Source: three-view drawing plus pictorial views. Frame: mm from the lowest corner of the part. A direction names the side the tool comes from. Give positions to 0.01 mm unless a question says otherwise; leave off trailing zeros. Write each loop counter-clockwise with the first axis right and the second up, starting at its lowest first coordinate (ties: lowest second). Pieces come first, ordered by that corner, then holes. Notation, with made-up numbers: M -22,87 L 31,87 A18 ccw 31,115 Z; hole C 20,35 d6. An arc over 180 degrees is marked long. One line per question, with ' | ' between items.
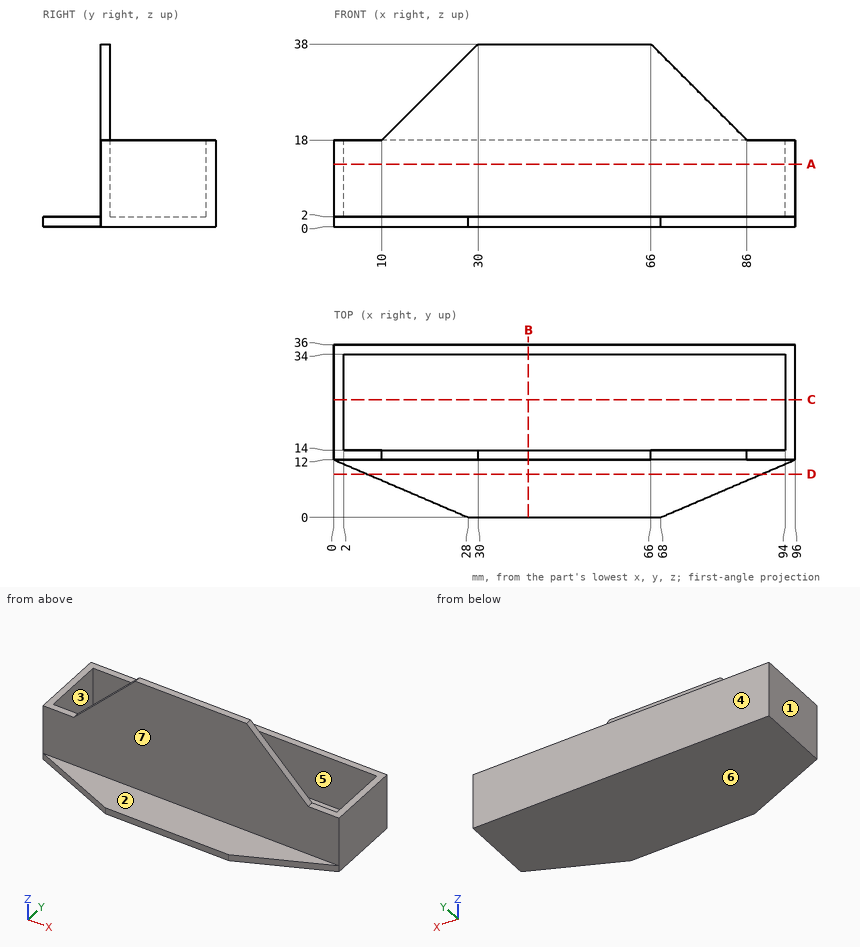
(1) Cut plane A-A, the plane z = 13. Return loops of the section in (x, y), then the cut area to 3 significant figures.
Working result:
outline: M 0,12 L 96,12 L 96,36 L 0,36 Z; hole M 2,14 L 94,14 L 94,34 L 2,34 Z | area: 464 mm^2
(2) Cut plane B-B, the plane x = 40.5. Return loops of the section in (y, z), then the cut area to 3 significant figures.
Working result:
outline: M 0,0 L 36,0 L 36,18 L 34,18 L 34,2 L 14,2 L 14,38 L 12,38 L 12,2 L 0,2 Z | area: 176 mm^2
(3) Material intervals for L1, parallel to X at y = 25, z = 15; L2, parallel to Y at x = 29.5, z = 11; L3, parallel to Z at x = 89.5, y = 33, sorted ascending. Write a range as [from, to].
Working result:
L1: x = [0, 2], [94, 96] | L2: y = [12, 14], [34, 36] | L3: z = [0, 2]
(4) Cut plane C-C, the plane y = 24.5. Return loops of the section in (x, z), then the cut area to 3 significant figures.
Working result:
outline: M 0,0 L 96,0 L 96,18 L 94,18 L 94,2 L 2,2 L 2,18 L 0,18 Z | area: 256 mm^2
(5) Cut plane D-D, the plane y = 9. Return loops of the section in (x, z).
Working result:
outline: M 7,0 L 89,0 L 89,2 L 7,2 Z
(6) First-contact query: P1, Ø8, axis at x = 26, z = 26, coming from the -Y side; P2, Ø1, axis at x = 41.5, z = 22.5, coming from the +Y side; P3, Ø10, axis at x = 34.5, y = 20.5, coming from the +Z side; P4, Ø10, axis at y = 30.5, z = 24.5, coming from the -X side. Flat tips, straight axial feed; report the tip coordinate or a pass-through.
Working result:
P1: stops at y = 12 | P2: stops at y = 14 | P3: stops at z = 2 | P4: passes through
(7) Draft query along Y for the marked faces 4, 5, 6 and 7. Return one class per face: released by +Y, released by -Y, zero draft, split by the parting line, or undercut.
Working result:
face 4: released by +Y | face 5: undercut | face 6: zero draft | face 7: released by -Y
(8) Set-up query: the marked faces 1, 2 and 3. Return all of +Z, -Z, +X, -X, +Y, -Y with unobstructed straight access to the full face (end or side cutting, diameter ignored); none if empty.
Working result:
face 1: +Z, -Z, -X, +Y, -Y | face 2: +Z, +X, -X, -Y | face 3: +Z
